```python
from build123d import *

# Parameters (mm, degrees)
SZKIC1_W                    = 220
SZKIC1_H                    = 74
SZKIC1_R                    = 6.5
DODANIE_WYCI_GNI_CIE1_DEPTH = 5


with BuildPart() as part:
    # Szkic1 → Dodanie-wyciągnięcie1 (new body)
    with BuildSketch(Plane(origin=(0, 0, 0), x_dir=(1, 0, 0), z_dir=(0, 1, 0))):
        with Locations((110, 37)):
            Rectangle(SZKIC1_W, SZKIC1_H)
        with Locations(Location((17.5, 37, 0), (0, 0, 270))):
            Circle(SZKIC1_R, mode=Mode.SUBTRACT)
        with Locations(Location((70.5, 37, 0), (0, 0, 270))):
            Circle(SZKIC1_R, mode=Mode.SUBTRACT)
        with Locations(Location((202.5, 37, 0), (0, 0, 90))):
            Circle(SZKIC1_R, mode=Mode.SUBTRACT)
        with Locations(Location((136.5, 37, 0), (0, 0, 90))):
            Circle(SZKIC1_R, mode=Mode.SUBTRACT)
        with Locations(Location((17.5, 17, 0), (0, 0, 270))):
            Circle(SZKIC1_R, mode=Mode.SUBTRACT)
        with BuildLine():
            ThreePointArc((17.5, 63.5), (11, 57), (17.5, 50.5))
            ThreePointArc((17.5, 50.5), (19.59786757, 50.434248184), (21.6875, 50.237250845))
            ThreePointArc((21.6875, 50.237250845), (28.949018821, 55.873769666), (23.3125, 63.135288487))
            ThreePointArc((23.3125, 63.135288487), (20.411965433, 63.408732555), (17.5, 63.5))
        make_face(mode=Mode.SUBTRACT)
    extrude(amount=DODANIE_WYCI_GNI_CIE1_DEPTH)


solid = part.part
```
Input: part model. Units: mm. Frame: model coordinates. A direction names the side the tool comes from. Give positions to 0.01 mm unless a question says otherwise; leave off trailing zeros. Write each loop counter-clockwise with the first axis right and the second up, starting at its lowest first coordinate (ties: lowest second). Pieces come first, ordered by that corner, then holes. Notation, with made-up numbers: (-9.5, -19.75) - (19.5, -19.75) arc R21 ccw to (19.5, -4.75) - close; hole circle Ø7 at (54.5, 53). An arc over 180 degrees is marked (long way). Write item = value, one per line. Start each with the question number.
1. Mould query, pull axis X, two halves, no side actions, for faces 1 (the cylindrical face through (140.455, 2.465, -31.842)), 2 (the cylindrical face through (28.93, 2.46, -55.73)), 3 (the flat face through (0, 2, -36)), 4 (the flat face through (220, 2, -36)). Classes: released by +X, released by -X, zero draft, split by the parting line, or undercut.
2. Section query D-D, the plane z = -36. Output: boundary loops of the cut face in (x, y), then the cut area to 3 significant figures.
3. Section query B-B, the plane x = 70.5. Output: boundary loops of the cut face in (y, z).
4. Section query C-C, the plane z = -14. Output: boundary loops of the cut face in (x, y).
5. Section query A-A, the plane y = 1.65. Output: boundary loops of the cut face in (x, z), then the cut area to 3 significant figures.
6. Ray query, L1, parallel to X at y = 2.65, z = -37; L2, parallel to Z at x = 202.5, y = 0.75; L3, parallel to Z at x = 20, y = 0.55. Return the intervals inside material, ascending.
7. Access query for faces 5 (the flat face through (108, 2, -74)), 6 (the cylindrical face through (20.453, 2.465, -63.406)). Directions: +Z, -Z, +X, -X, +Y, -Y. A direction counts if a zero-diameter tool reaches every point of the face in a straight line with its end or side. Return the directions, or none.
Check sheet entries:
q1.face_1 = undercut
q1.face_2 = undercut
q1.face_3 = released by -X
q1.face_4 = released by +X
q2.outline = (0, 0) - (11.08, 0) - (11.08, 5) - (0, 5) - close; (23.92, 0) - (64.08, 0) - (64.08, 5) - (23.92, 5) - close; (76.92, 0) - (130.08, 0) - (130.08, 5) - (76.92, 5) - close; (142.92, 0) - (196.08, 0) - (196.08, 5) - (142.92, 5) - close; (208.92, 0) - (220, 0) - (220, 5) - (208.92, 5) - close
q2.area = 843 mm2
q3.outline = (0, -74) - (5, -74) - (5, -43.5) - (0, -43.5) - close; (0, -30.5) - (5, -30.5) - (5, 0) - (0, 0) - close
q4.outline = (0, 0) - (11.73, 0) - (11.73, 5) - (0, 5) - close; (23.27, 0) - (220, 0) - (220, 5) - (23.27, 5) - close
q5.outline = (0, -74) - (220, -74) - (220, 0) - (0, 0) - close; hole circle Ø13 at (17.5, -37); hole circle Ø13 at (17.5, -17); hole (17.5, -63.5) arc R46.5 ccw to (23.31, -63.14) arc R6.5 ccw to (21.69, -50.24) arc R33.5 cw to (17.5, -50.5) arc R6.5 ccw to start; hole circle Ø13 at (70.5, -37); hole circle Ø13 at (136.5, -37); hole circle Ø13 at (202.5, -37)
q5.area = 15,400 mm2
q6.L1 = 0 to 11, 24 to 64, 77 to 130, 143 to 196, 209 to 220
q6.L2 = -74 to -43.5, -30.5 to 0
q6.L3 = -74 to -63.43, -50.41 to -43, -31 to -23, -11 to 0
q7.face_5 = -Z, +X, -X, +Y, -Y
q7.face_6 = +Y, -Y
